Work out the finished part from the listing and answer in its coordinate system (mm). A direction names the side the tool comes from. Coordinates: 2 decimals unless noted, no trailing zeros. Order: outer loops, then holes, each group sorted by start corner. A loop starts at its lowest first (then second) coordinate and runs counter-clockwise, first axis right, second up. Notation, with made-up numbers: M 26.5,-30.5 L 46.5,-30.5 A25 cw 46.5,-11.5 Z; hole C -37,71 d6. An arc over 180 degrees is marked long. Answer in a Markdown table with one row per item. Add a question column.
Item 1: Consider line 1 (X direction, y = 0.85, z = 0); line 2 (Z direction, x = -1, y = 0.9); line 3 (X direction, y = 2.2, z = 18.5). Determine where each line is inside the solid, lowest interval first. Write a range as from..to.
Item 2: Which of the six approach directions +Z, -Z, +X, -X, +Y, -Y give full straight-line access (tool end or side, diameter ignored) to faces 5 (the face through (18, 1, 4)), 6 (the face through (4, 1, -18)), 7 (the face through (7.94, 0.89, -0.35))?
Item 3: The part is cut by section B-B (z = -12.5). Write down the section's boundary in (x, y), then the cut area to 3 significant figures.
Item 4: The part is cut by section C-C (x = -18). Write down the section's boundary in (y, z), then the cut area to 3 significant figures.
Item 5: Flat-ended cylindrical pins translate along their axes: pin 1 Ø0.9 at (y, z) = (2, 19.5) entering from -X; pin 2 Ø1.9 at (x, z) = (0, 22) entering from -Y; pin 3 Ø1.5 at (x, y) = (17, 2) entering from -Z; pin 4 Ø5 at (x, z) = (0, -12.5) entering from +Y. Find the tip coordinate at first contact, or state that the pin passes through.
Item 6: The mould has two halves that part along X. Classify faces 1 (the face through (0, 1, -26)), 2 (the face through (18, 1, -4)), 3 (the face through (0.07, 0.89, -14.1)), 4 (the face through (0.07, 0.89, 10.9)): released by +X, released by -X, zero draft, split by the parting line, or undercut.
Item 7: The part is cut by section A-A (y = 1.15). State how many separate pieces and enclosed holes the cut face has, then the cut area to 3 significant figures.
Item 8: The part is cut by section D-D (z = -21). Write down the section's boundary in (x, y), then the cut area to 3 significant figures.
from build123d import *

# Parameters (mm, degrees)
BOSS_EXTRUDE1_DEPTH = 3
SKETCH2_R           = 1.6
CUT_EXTRUDE1_DEPTH  = 25
CHAMFER1_SIZE       = 1.25
FILLET1_R           = 10
SKETCH3_R           = 5.7
CUT_EXTRUDE2_DEPTH  = 3


with BuildPart() as part:
    # Sketch1 → Boss-Extrude1 (new body)
    with BuildSketch(Plane(origin=(0, 0, 0), x_dir=(1, 0, 0), z_dir=(0, 1, 0))):
        Polygon((4, 4), (4, 22), (-4, 22), (-4, 4), (-22, 4), (-22, -4), (-4, -4), (-4, -22), (4, -22), (4, -4), (22, -4), (22, 4), align=None)
        with BuildLine():
            ThreePointArc((-4, 22), (0, 26), (4, 22))
            Line((4, 22), (-4, 22))
        make_face()
        with BuildLine():
            ThreePointArc((22, 4), (26, 0), (22, -4))
            Line((22, -4), (22, 4))
        make_face()
        with BuildLine():
            Line((-22, 4), (-22, -4))
            ThreePointArc((-22, -4), (-26, 0), (-22, 4))
        make_face()
        with BuildLine():
            ThreePointArc((4, -22), (0, -26), (-4, -22))
            Line((-4, -22), (4, -22))
        make_face()
    extrude(amount=BOSS_EXTRUDE1_DEPTH)

    # Sketch2 → Cut-Extrude1 (cut)
    with BuildSketch(Plane(origin=(0, 3, 0), x_dir=(1, 0, 0), z_dir=(0, 1, 0))):
        with Locations(Location((-22, 0, 0), (0, 0, 270))):
            Circle(SKETCH2_R)
        with Locations(Location((0, 22, 0), (0, 0, 270))):
            Circle(SKETCH2_R)
        with Locations(Location((0, -22, 0), (0, 0, 270))):
            Circle(SKETCH2_R)
        with Locations(Location((22, 0, 0), (0, 0, 270))):
            Circle(SKETCH2_R)
        with Locations(Location((0, 12.5, 0), (0, 0, 270))):
            Circle(SKETCH2_R)
        with Locations(Location((-9.5, 0, 0), (0, 0, 270))):
            Circle(SKETCH2_R)
        with Locations(Location((0, -12.5, 0), (0, 0, 270))):
            Circle(SKETCH2_R)
        with Locations(Location((9.5, 0, 0), (0, 0, 270))):
            Circle(SKETCH2_R)
    extrude(amount=-CUT_EXTRUDE1_DEPTH, mode=Mode.SUBTRACT)

    # Chamfer1
    chamfer1_edges = [part.edges().sort_by_distance(p)[0] for p in [
        (9.5, 3, -1.6),
        (0, 3, 10.9),
        (-9.5, 3, -1.6),
        (0, 3, -14.1),
    ]]
    chamfer(chamfer1_edges, length=CHAMFER1_SIZE)

    # Fillet1
    fillet1_edges = [part.edges().sort_by_distance(p)[0] for p in [
        (4, 1.5, -4),
        (4, 1.5, 4),
        (-4, 1.5, 4),
        (-4, 1.5, -4),
    ]]
    fillet(fillet1_edges, radius=FILLET1_R)

    # Sketch3 → Cut-Extrude2 (cut)
    with BuildSketch(Plane(origin=(0, 3, 0), x_dir=(1, 0, 0), z_dir=(0, 1, 0))):
        with Locations(Location((0, 0, 0), (0, 0, 270))):
            Circle(SKETCH3_R)
    extrude(amount=-CUT_EXTRUDE2_DEPTH, mode=Mode.SUBTRACT)


solid = part.part
Reply:
| question | item | result |
|---|---|---|
| 1 | line 1 | x = -26..-23.6, -20.4..-11.1, -7.9..-5.7, 5.7..7.9, 11.1..20.4, 23.6..26 |
| 1 | line 2 | z = -25.87..-23.25, -20.75..-13.75, -11.25..-5.61, 5.61..11.25, 13.75..20.75, 23.25..25.87 |
| 1 | line 3 | x = -4..4 |
| 2 | face 5 | +Z, +X, +Y, -Y |
| 2 | face 6 | -Z, +X, +Y, -Y |
| 2 | face 7 | +Y, -Y |
| 3 | outline | M -4.11,0 L -1.6,0 L -1.6,1.75 L -2.85,3 L -4.11,3 Z; M 1.6,0 L 4.11,0 L 4.11,3 L 2.85,3 L 1.6,1.75 Z |
| 3 | area | 13.5 mm2 |
| 4 | outline | M 0,-4 L 3,-4 L 3,4 L 0,4 Z |
| 4 | area | 24.0 mm2 |
| 5 | pin 1 | stops at x = -4 |
| 5 | pin 2 | passes through |
| 5 | pin 3 | stops at z = -4 |
| 5 | pin 4 | stops at y = 2.65 |
| 6 | face 1 | split by the parting line |
| 6 | face 2 | zero draft |
| 6 | face 3 | undercut |
| 6 | face 4 | undercut |
| 7 | separate pieces | 1 |
| 7 | enclosed holes | 9 |
| 7 | area | 660 mm2 |
| 8 | outline | M -4,0 L -1.25,0 L -1.25,3 L -4,3 Z; M 1.25,0 L 4,0 L 4,3 L 1.25,3 Z |
| 8 | area | 16.5 mm2 |
